Design review of the part built by this model. Coordinates are the model's own, in mm. A direction names the side the tool comes from. Round coordinates to 2 decimals unless told otherwise and drop trailing zeros. Order: outer loops, then holes, each group sorted by start corner. A loop starts at its lowest first (then second) coordinate and runs counter-clockwise, first axis right, second up.
from build123d import *

# Parameters (mm, degrees)
BOSS_EXTRUDE1_DEPTH   = 2
SKETCH2_W             = 2.5
SKETCH2_H             = 5
BOSS_EXTRUDE2_DEPTH   = 15
SKETCH5_W             = 15
SKETCH5_H             = 2
BOSS_EXTRUDE3_DEPTH   = 10
CHAMFER1_SIZE         = 10
CHAMFER1_SIZE2        = 2.679491924
CHAMFER1_PART_2_SIZE  = 10
CHAMFER1_PART_2_SIZE2 = 2.679491924
SKETCH6_R             = 1.25
CUT_EXTRUDE1_DEPTH    = 18
SKETCH7_R             = 1.75
CUT_EXTRUDE2_DEPTH    = 3
CUT_EXTRUDE3_DEPTH    = 20


with BuildPart() as part:
    # Sketch1 → Boss-Extrude1 (new body)
    with BuildSketch(Plane.XY):
        Polygon((23, 10.5), (-23, 10.5), (-23, -10.5), (-7.5, -10.5), (-7.5, -5.5), (7.5, -5.5), (7.5, -10.5), (23, -10.5), align=None)
    extrude(amount=BOSS_EXTRUDE1_DEPTH)

    # Sketch2 → Boss-Extrude2 (add)
    with BuildSketch(Plane.XY.offset(2)):
        with Locations((-8.75, -8)):
            Rectangle(SKETCH2_W, SKETCH2_H)
        with Locations((8.75, -8)):
            Rectangle(SKETCH2_W, SKETCH2_H)
    extrude(amount=BOSS_EXTRUDE2_DEPTH)

    # Sketch5 → Boss-Extrude3 (add)
    with BuildSketch(Plane.XY.offset(17)):
        with Locations((0, -9.5)):
            Rectangle(SKETCH5_W, SKETCH5_H)
    extrude(amount=-BOSS_EXTRUDE3_DEPTH)

    # Chamfer1
    chamfer1_edges = [part.edges().sort_by_distance(p)[0] for p in [
        (-8.75, -5.5, 17),
    ]]
    chamfer1_side = [part.faces().sort_by_distance(p)[0] for p in [
        (-8.75, -5.5, 9.5),
    ]]
    chamfer(chamfer1_edges, length=CHAMFER1_SIZE, length2=CHAMFER1_SIZE2, reference=chamfer1_side[0])

    # Chamfer1 part 2
    chamfer1_part_2_edges = [part.edges().sort_by_distance(p)[0] for p in [
        (8.75, -5.5, 17),
    ]]
    chamfer1_part_2_side = [part.faces().sort_by_distance(p)[0] for p in [
        (8.75, -5.5, 9.5),
    ]]
    chamfer(chamfer1_part_2_edges, length=CHAMFER1_PART_2_SIZE, length2=CHAMFER1_PART_2_SIZE2, reference=chamfer1_part_2_side[0])

    # Sketch6 → Cut-Extrude1 (cut, through all)
    with BuildSketch(Plane(origin=(0, 0, 0), x_dir=(-1, 0, 0), z_dir=(0, 0, -1))):
        with Locations((21, 8.5)):
            Circle(SKETCH6_R)
        with Locations((-21, -8.5)):
            Circle(SKETCH6_R)
        with Locations((-21, 8.5)):
            Circle(SKETCH6_R)
        with Locations((21, -8.5)):
            Circle(SKETCH6_R)
    extrude(amount=-CUT_EXTRUDE1_DEPTH, mode=Mode.SUBTRACT)

    # Sketch7 → Cut-Extrude2 (cut, through all)
    with BuildSketch(Plane(origin=(0, -8.5, 0), x_dir=(1, 0, 0), z_dir=(0, 1, 0))):
        with Locations((-5, -12.755907313)):
            Circle(SKETCH7_R)
        with Locations((5, -12.755907313)):
            Circle(SKETCH7_R)
    extrude(amount=-CUT_EXTRUDE2_DEPTH, mode=Mode.SUBTRACT)

    # Sketch8 → Cut-Extrude3 (cut, through all)
    with BuildSketch(Plane(origin=(0, -8.5, 0), x_dir=(1, 0, 0), z_dir=(0, 1, 0))):
        Polygon((5, -16.220008928), (8, -14.487958121), (8, -11.023856505), (5, -9.291805698), (2, -11.023856505), (2, -14.487958121), align=None)
        Polygon((-5, -16.220008928), (-2, -14.487958121), (-2, -11.023856505), (-5, -9.291805698), (-8, -11.023856505), (-8, -14.487958121), align=None)
    extrude(amount=CUT_EXTRUDE3_DEPTH, mode=Mode.SUBTRACT)


solid = part.part
1) Take a section at D-D on y = 5.5. Give the boundary of the cut face in (x, z).
Results:
outline: (-23, 0) - (23, 0) - (23, 2) - (-23, 2) - close
2) Take a section at A-A on z = 6.5. Give the boundary of the cut face in (x, y), plus the area to 3 significant figures.
Results:
outline: (-10, -10.5) - (-7.5, -10.5) - (-7.5, -5.5) - (-10, -5.5) - close; (7.5, -10.5) - (10, -10.5) - (10, -5.5) - (7.5, -5.5) - close
area: 25.0 mm2
3) Take a section at C-C on x = 9.5. Give the boundary of the cut face in (y, z), plus the area to 3 significant figures.
Results:
outline: (-10.5, 0) - (10.5, 0) - (10.5, 2) - (-5.5, 2) - (-5.5, 7) - (-8.18, 17) - (-10.5, 17) - close
area: 104 mm2
4) For faces 1 (the face through (7.5, -8, 4)), 2 (the face through (7.5, -8.1, 15.6)), 3 (the face through (-9, -5.5, 4)), list the 3-axis set-ups (+Z, -Z, +X, -X, +Y, -Y) from which the entire face can be reached by the end or side of a thin tool; tool diameter is ignored.
Results:
face 1: -Z
face 2: +Z, -Z, +Y
face 3: +Z, +X, -X, +Y
5) The part is to be moulded in two halves that separate along X. For faces 4 (the face through (0, -9, 17)), 5 (the face through (0, -5.5, 1)), 6 (the face through (10, -9, 8)), say which applies: released by +X, released by -X, zero draft, split by the parting line, or undercut.
Results:
face 4: zero draft
face 5: undercut
face 6: released by +X
6) Take a section at B-B on x = -5. Give the boundary of the cut face in (y, z), plus the area to 3 significant figures.
Results:
outline: (-10.5, 7) - (-8.5, 7) - (-8.5, 11.01) - (-10.5, 11.01) - close; (-10.5, 14.51) - (-8.5, 14.51) - (-8.5, 17) - (-10.5, 17) - close; (-5.5, 0) - (10.5, 0) - (10.5, 2) - (-5.5, 2) - close
area: 45.0 mm2
7) To check wall thickness, follow line 1 along Y through (x, z) = (-21, 0.4); line 2 along X through (y, z) = (-7, 1); line 3 along Y through (x, z) = (9, 6.75). State the ranges of each line that lie inside material, in increasing order.
Results:
line 1: y = -10.5 to -9.75, -7.25 to 7.25, 9.75 to 10.5
line 2: x = -23 to -7.5, 7.5 to 23
line 3: y = -10.5 to -5.5
8) Clearance check with flat-ended pins moving along their axes: P1, Ø5.5, axis at y = -7.5, z = 10.5, coming from the -X side; P2, Ø4.5, axis at x = 5, z = 12.76, coming from the -Y side; P3, Ø6.5, axis at x = -10.5, y = 4.5, coming from the +Z side; P4, Ø5, axis at x = -11, z = 7.5, coming from the +Y side. State where each tip first meets the part, or that it passes through.
Results:
P1: stops at x = -10
P2: stops at y = -10.5
P3: stops at z = 2
P4: stops at y = -5.5
